Geometry check sheet. Reference: the model listing, model coordinates, mm. A direction names the side the tool comes from. Give positions to 0.01 mm unless a question says otherwise; leave off trailing zeros. Loops run counter-clockwise (first coordinate to the right, second up) from the corner with the lowest first, then second, coordinate; pieces in that order, holes last. Notation, with made-up numbers: (53, 53.25) -> (64, 53.25) arc R23 ccw to (64, 92.25) -> close; hole circle Ø1 at (8, -37.5). An arc over 180 degrees is marked (long way). Answer as a JSON object with one key per item and string values.
from build123d import *

# Parameters (mm, degrees)
SKETCH1_W                  = 35
SKETCH1_H                  = 50
BOSS_EXTRUDE1_DEPTH        = 40
CHAMFER1_SIZE              = 1
M8_TAPPED_HOLE1_AT_2_COUNT = 2
M8_TAPPED_HOLE1_AT_2_PITCH = 40.311288741


with BuildPart() as part:
    # Sketch1 → Boss-Extrude1 (new body)
    with BuildSketch(Plane(origin=(0, 0, 0), x_dir=(1, 0, 0), z_dir=(0, 1, 0))):
        Rectangle(SKETCH1_W, SKETCH1_H)
    extrude(amount=-BOSS_EXTRUDE1_DEPTH)

    # Chamfer1
    chamfer1_edges = [part.edges().sort_by_distance(p)[0] for p in [
        (-17.5, -40, 0),
        (0, -40, 25),
        (17.5, -40, 0),
        (0, 0, 25),
        (-17.5, 0, 0),
        (0, 0, -25),
        (17.5, 0, 0),
        (17.5, -20, 25),
        (-17.5, -20, 25),
        (-17.5, -20, -25),
        (17.5, -20, -25),
        (0, -40, -25),
    ]]
    chamfer(chamfer1_edges, length=CHAMFER1_SIZE)

    # Sketch3 → M8 Tapped Hole1 (revolve, cut)
    with BuildSketch(Plane(origin=(-10, 0, -17.5), x_dir=(0, 0, 1), z_dir=(1, 0, 0))):
        Polygon((0, 0), (0, 21.792926105), (3.4, 19.75), (3.4, 0), align=None)
    m8_tapped_hole1 = revolve(axis=Axis((-10, 6.35, -17.5), (0, -1, 0)), mode=Mode.SUBTRACT)

    # M8 Tapped Hole1 at 2: M8 Tapped Hole1 ×2
    with Locations(*[Vector(0.4961389383568339, 0, 0.8682431421244592) * (i * M8_TAPPED_HOLE1_AT_2_PITCH) for i in range(1, M8_TAPPED_HOLE1_AT_2_COUNT)]):
        add(m8_tapped_hole1, mode=Mode.SUBTRACT)

    # Mirror1: M8 Tapped Hole1 across plane
    add(m8_tapped_hole1.mirror(Plane.XY), mode=Mode.SUBTRACT)

    # Mirror1 copy 1 sketch → Mirror1 copy 1 (revolve, cut)
    with BuildSketch(Plane(origin=(10, 0, -17.5), x_dir=(0, 0, -1), z_dir=(1, 0, 0))):
        Polygon((0, 0), (0, -21.792926105), (3.4, -19.75), (3.4, 0), align=None)
    revolve(axis=Axis((10, 6.35, -17.5), (0, 1, 0)), mode=Mode.SUBTRACT)


solid = part.part
1) Section check A-A on y = -15.5. Record the cut outline in (x, z), plus the area to 3 significant figures.
Geometry check:
{"outline": "(-17.5, -24) -> (-16.5, -25) -> (16.5, -25) -> (17.5, -24) -> (17.5, 24) -> (16.5, 25) -> (-16.5, 25) -> (-17.5, 24) -> close; hole circle Ø6.8 at (-10, -17.5); hole circle Ø6.8 at (-10, 17.5); hole circle Ø6.8 at (10, -17.5); hole circle Ø6.8 at (10, 17.5)", "area": "1,600 mm2"}
2) Draft check along X on faces 1 (the face through (17.5, -20, 0)), 2 (the face through (0, -40, 0)), 3 (the face through (10.359, -21.438, -17.031)), 4 (the face through (-17.5, -20, 0)). Enter one of: pulls with the +X half, pulls with the -X half, needs draft (parallel to the pull), parting line crosses it, or undercut.
Geometry check:
{"face 1": "pulls with the +X half", "face 2": "needs draft", "face 3": "undercut", "face 4": "pulls with the -X half"}
3) Tool access check on faces 5 (the face through (0, -20, -25)), 6 (the face through (-6.68, -9.74, 18.24)). Record the directions out of +Z, -Z, +X, -X, +Y, -Y that give a thin tool (end or side, any length) a straight path to the whole face; none if there is none.
Geometry check:
{"face 5": "-Z, +X, -X, +Y, -Y", "face 6": "+Y"}
4) Material ranges on line 1 along X through (y, z) = (-10, -17.5); line 2 along Z through (x, y) = (10, -15); line 3 along X through (y, z) = (-18, -20), recorded low to high. Write a range as from..to.
Geometry check:
{"line 1": "x = -17.5..-13.4, -6.6..6.6, 13.4..17.5", "line 2": "z = -25..-20.9, -14.1..14.1, 20.9..25", "line 3": "x = -17.5..-12.3, -7.7..7.7, 12.3..17.5"}
